Verification items for the finished model (mm, model axes). Round coordinates to 2 decimals unless told otherwise and drop trailing zeros. Write each loop counter-clockwise with the first axis right and the second up, starting at its lowest first coordinate (ties: lowest second). Pieces come first, ordered by that corner, then holes. Notation, with made-up numbers: (77.25, 30) -> (135.25, 30) arc R28 ccw to (135.25, 68) -> close; hole circle Ø7 at (55.25, 34). An arc over 180 degrees is marked (long way). Answer as a JSON object with one key per item and string values. Group by question number.
(1) Scan lines: L1, parallel to Z at x = -10.65, y = 2.2; L2, parallel to X at y = 0.45, z = 11; L3, parallel to Z at x = -11, y = 1.85. Record each from-to range of solid material in increasing order. Write a range as from..to.
(2) Sectioned sample at C-C on y = 2. Record the cut outline in (x, z).
(3) Sectioned sample at A-A on z = 35. Record the cut outline in (x, y).
(4) Sectioned sample at D-D on z = 50. Record the cut outline in (x, y).
(5) Sectioned sample at B-B on x = -10.65. Record the cut outline in (y, z), and give its area (3 significant figures).
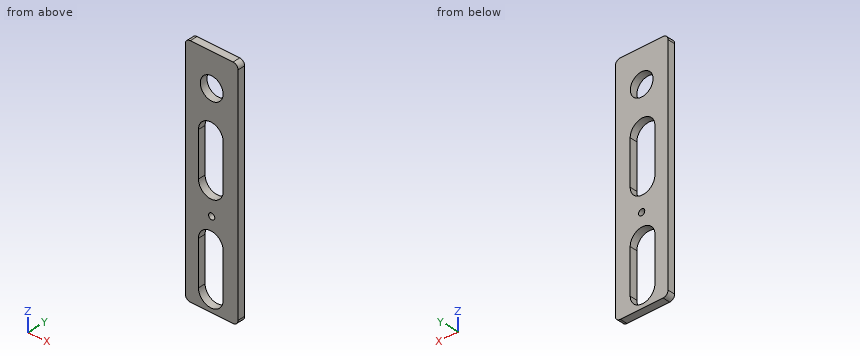
Autodesk Inventor part; units mm, degrees
ref_plane "YZ Plane" through (0, 0, 0) normal (1, 0, 0) x (0, 1, 0)
ref_plane "XZ Plane" through (0, 0, 0) normal (0, 1, 0) x (-1, 0, 0)
ref_plane "XY Plane" through (0, 0, 0) normal (0, 0, 1) x (1, 0, 0)
sketch "Sketch1" plane through (0, 0, 0) normal (0, 1, 0) x (-1, 0, 0)
  line L0 (2, 0) -> (19.3, 0)
  line L1 (21.3, 2) -> (21.3, 93)
  line L2 (19.3, 95) -> (2, 95)
  line L3 (0, 93) -> (0, 2)
  circle A0 centre (10.65, 35) radius 1.25
  arc A1 (21.3, 93) -> (19.3, 95) centre (19.3, 93) ccw
  arc A2 (2, 95) -> (0, 93) centre (2, 93) ccw
  arc A3 (0, 2) -> (2, 0) centre (2, 2) ccw
  arc A4 (19.3, 0) -> (21.3, 2) centre (19.3, 2) ccw
  circle A5 centre (10.65, 81.5) radius 4.6
  line L4 (11, 46.1899) -> (11, 64.1899) construction
  line L5 (6, 46.1899) -> (6, 64.1899)
  line L6 (16, 64.1899) -> (16, 46.1899)
  arc A6 (6, 46.1899) -> (16, 46.1899) centre (11, 46.1899) ccw
  arc A7 (16, 64.1899) -> (6, 64.1899) centre (11, 64.1899) ccw
  line L7 (11, 6.6463) -> (11, 24.6463) construction
  line L8 (6, 6.6463) -> (6, 24.6463)
  line L9 (16, 24.6463) -> (16, 6.6463)
  arc A8 (6, 6.6463) -> (16, 6.6463) centre (11, 6.6463) ccw
  arc A9 (16, 24.6463) -> (6, 24.6463) centre (11, 24.6463) ccw
  point P0 (0, 0)
  point P1 (21.3, 95)
  point P2 (21.3, 0)
  point P3 (11, 55.1899)
  point P4 (11, 15.6463)
  dimension "d0" = 21.3
  dimension "d1" = 95
  dimension "d2" = 2.5
  dimension "d3" = 35
  dimension "d6" = 10.65
  dimension "d8" = 2
  dimension "d9" = 9.2
  dimension "d10" = 46.5
  dimension "d13" = 18
  dimension "d14" = 5
  dimension "d17" = 11.1898
  dimension "d18" = 18
  dimension "d19" = 5
extrude "Extrusion1" add sketch "Sketch1" along normal blind 3 contours A3 L3 A2 L2 A1 L1 A4 L0 | L5 A7 L6 A6 | L8 A9 L9 A8
extrude "Extrusion2" cut sketch "Sketch1" along normal through all contours L5 A7 L6 A6 | L8 A9 L9 A8
equation "\"d6\" = 0.5 * d0"
equation "\"d19\" = d14"
properties part number "12mero"
Computed values:
{
 "1": {"L1": "0..1.66, 29.63..33.75, 36.25..41.2, 69.18..76.9, 86.1..95", "L2": "-21.3..-16, -6..0", "L3": "0..1.65, 29.65..33.8, 36.2..41.19, 69.19..76.91, 86.09..95"},
 "2": {"outline": "(-21.3, 2) arc R2 ccw to (-19.3, 0) -> (-2, 0) arc R2 ccw to (0, 2) -> (0, 93) arc R2 ccw to (-2, 95) -> (-19.3, 95) arc R2 ccw to (-21.3, 93) -> close; hole (-16, 6.65) arc R5 ccw to (-6, 6.65) -> (-6, 24.65) arc R5 ccw to (-16, 24.65) -> close; hole (-16, 46.19) arc R5 ccw to (-6, 46.19) -> (-6, 64.19) arc R5 ccw to (-16, 64.19) -> close; hole circle Ø9.2 at (-10.65, 81.5); hole circle Ø2.5 at (-10.65, 35)"},
 "3": {"outline": "(-21.3, 0) -> (-11.9, 0) -> (-11.9, 3) -> (-21.3, 3) -> close; (-9.4, 0) -> (0, 0) -> (0, 3) -> (-9.4, 3) -> close"},
 "4": {"outline": "(-21.3, 0) -> (-16, 0) -> (-16, 3) -> (-21.3, 3) -> close; (-6, 0) -> (0, 0) -> (0, 3) -> (-6, 3) -> close"},
 "5": {"outline": "(0, 0) -> (3, 0) -> (3, 1.66) -> (0, 1.66) -> close; (0, 29.63) -> (3, 29.63) -> (3, 33.75) -> (0, 33.75) -> close; (0, 36.25) -> (3, 36.25) -> (3, 41.2) -> (0, 41.2) -> close; (0, 69.18) -> (3, 69.18) -> (3, 76.9) -> (0, 76.9) -> close; (0, 86.1) -> (3, 86.1) -> (3, 95) -> (0, 95) -> close", "area": "82.0 mm2"}
}
